Read the model definition and answer for the solid it produces. Units are mm, in the model's axes. A direction names the side the tool comes from. Coordinates: 2 decimals unless noted, no trailing zeros. Write each loop counter-clockwise with the first axis right and the second up, starting at its lowest first coordinate (ties: lowest second). Pieces come first, ordered by that corner, then holes. Notation, with made-up numbers: (-33.5, 4.5) -> (5.5, 4.5) arc R23 ccw to (5.5, 21.5) -> close; hole circle Ø1 at (77.25, -15). An arc over 180 degrees is marked (long way). Answer in a Markdown table with one row per item. Add a question column.
Item 1: Section D-D on x = 48.75 is taken. Write down the section's boundary in (y, z).
Item 2: Which of the six approach directions +Z, -Z, +X, -X, +Y, -Y give full straight-line access (tool end or side, diameter ignored) to faces 4 (the face through (56, 107, 18)), 5 (the face through (55.8, 105.5, 24))?
Item 3: For a pull along Y with two mould halves and no side action, classify faces 1 (the face through (56.175, 93.203, 22.859)), 2 (the face through (68.5, 101, 14)), 3 (the face through (55.811, 94.062, 12.93)) as +Y half, -Y half, draft (parallel to the pull), parting line (faces both ways), or undercut.
Item 4: Given pin 1 Ø1.7 at (x, y) = (56, 95.5) entering from +Z; pin 2 Ø1.2 at (x, y) = (55.5, 95.5) entering from -Z, each flat-ended and moving along its own axis, determine where each tip first touches the part or whether it passes through.
Item 5: Section A-A on z = 16 is taken. Write down the section's boundary in (x, y).
Item 6: Section C-C on z = 23 is taken. Write down the section's boundary in (x, y).
Item 7: Straight lines are drawn through the part: line 1 (Y direction, x = 56, z = 14.5); line 2 (X direction, y = 106.5, z = 15.5); line 3 (Y direction, x = 58.5, z = 19.75). For each, find the intervals that lie inside material, in ascending order. Write a range as from..to.
Item 8: Section B-B on x = 56 is taken. Write down the section's boundary in (y, z), then the cut area to 3 significant figures.
```python
from build123d import *

# Parameters (mm, degrees)
CYLINDER_R           = 5
CYLINDER_DEPTH       = 200
CYLINDER_PITCH_ANGLE = 90
BOX004_W             = 25
BOX004_H             = 18
BOX004_DEPTH         = 16
SKETCH005_R          = 1.45
POCKET005_DEPTH      = 10
FILLET001_R          = 4
CHAMFER003_SIZE      = 1


with BuildPart() as cylinder:
    # Cylinder → Cylinder (new body)
    with BuildSketch(Plane.XY):
        Circle(CYLINDER_R)
    extrude(amount=CYLINDER_DEPTH)


with BuildPart() as cylinder_1:
    # Cylinder pitch: moved
    add(cylinder.part.rotate(Axis((0, 0, 0), (0, 1, 0)), CYLINDER_PITCH_ANGLE))


with BuildPart() as cylinder_2:
    # Cylinder placement: moved
    add(cylinder_1.part.moved(Location((0, 121, 20))))


with BuildPart() as chamfer003:
    # Box004 → Box004 (new body)
    with BuildSketch(Plane(origin=(43.5, 112, 8), x_dir=(1, 0, 0), z_dir=(0, 0, 1))):
        with Locations((12.5, 9)):
            Rectangle(BOX004_W, BOX004_H)
    extrude(amount=BOX004_DEPTH)

    # Sketch005 → Pocket005 (cut)
    with BuildSketch(Plane(origin=(43.5, 112, 8), x_dir=(1, 0, 0), z_dir=(0, 0, -1))):
        with Locations((12.5, -3.5)):
            Circle(SKETCH005_R)
        with Locations((12.5, -14.5)):
            Circle(SKETCH005_R)
    extrude(amount=-POCKET005_DEPTH, mode=Mode.SUBTRACT)

    # Cut: cut Cylinder
    add(cylinder_2.part, mode=Mode.SUBTRACT)


with BuildPart() as chamfer003_1:
    # Cut placement: moved
    add(chamfer003.part.moved(Location((0, -20, 0))))

    # Fillet001
    fillet001_edges = [chamfer003_1.edges().sort_by_distance(p)[0] for p in [
        (56, 110, 24),
        (56, 92, 24),
    ]]
    fillet(fillet001_edges, radius=FILLET001_R)

    # Chamfer003
    chamfer003_edges = [chamfer003_1.edges().sort_by_distance(p)[0] for p in [
        (56, 104, 24),
        (56, 98, 24),
    ]]
    chamfer(chamfer003_edges, length=CHAMFER003_SIZE)


solid = chamfer003_1.part
```
Results below:
| question | item | result |
|---|---|---|
| 1 | outline | (92, 8) -> (110, 8) -> (110, 20) arc R4 ccw to (106, 24) -> (105, 24) -> (104.74, 23.32) arc R5 cw (long way) to (97.26, 23.32) -> (97, 24) -> (96, 24) arc R4 ccw to (92, 20) -> close |
| 2 | face 4 | -Z |
| 2 | face 5 | +Z, +X, -X, +Y, -Y |
| 3 | face 1 | -Y half |
| 3 | face 2 | draft |
| 3 | face 3 | undercut |
| 4 | pin 1 | stops at z = 24 |
| 4 | pin 2 | stops at z = 18 |
| 5 | outline | (43.5, 92) -> (68.5, 92) -> (68.5, 98) -> (43.5, 98) -> close; (43.5, 104) -> (68.5, 104) -> (68.5, 110) -> (43.5, 110) -> close; hole circle Ø2.9 at (56, 95.5); hole circle Ø2.9 at (56, 106.5) |
| 6 | outline | (43.5, 93.35) -> (68.5, 93.35) -> (68.5, 97) -> (43.5, 97) -> close; (43.5, 105) -> (68.5, 105) -> (68.5, 108.65) -> (43.5, 108.65) -> close |
| 7 | line 1 | y = 92..94.05, 96.95..105.05, 107.95..110 |
| 7 | line 2 | x = 43.5..54.55, 57.45..68.5 |
| 7 | line 3 | y = 92..96.01, 105.99..110 |
| 8 | outline | (92, 8) -> (94.05, 8) -> (94.05, 18) -> (96.42, 18) arc R5 cw to (97.26, 23.32) -> (97, 24) -> (96, 24) arc R4 ccw to (92, 20) -> close; (96.95, 8) -> (105.05, 8) -> (105.05, 17.07) arc R5 cw to (96.95, 17.07) -> close; (104.74, 23.32) arc R5 cw to (105.58, 18) -> (107.95, 18) -> (107.95, 8) -> (110, 8) -> (110, 20) arc R4 ccw to (106, 24) -> (105, 24) -> close |
| 8 | area | 149 mm2 |
